The model under review builds one solid part; all positions refer to its coordinate system, in mm. A direction names the side the tool comes from. Round coordinates to 2 decimals unless told otherwise and drop trailing zeros. Write each loop counter-clockwise with the first axis right and the second up, starting at its lowest first coordinate (ties: lowest second). Pieces come first, ordered by that corner, then holes. Notation, with made-up numbers: M 1.25,88.25 L 53.25,88.25 A22 cw 53.25,114.25 Z; hole C 84,-37.5 d2. An arc over 180 degrees is marked long. One line per item, written item: value. Start each with the question number.
1) Take a section at B-B, the plane z = 10. Write out the cut boundary in (x, y).
2) Wall thickness on probe 1 along X at (y, z) = (0, 4.25); probe 2 along Z at (x, y) = (1.5, -5.5): over which ranges is each line inside the solid? List them lowest first.
3) Take a section at C-C, the plane y = 0. Write out the cut boundary in (x, z), and give its area (3 significant figures).
4) Take a section at D-D, the plane z = 4.25. Write out the cut boundary in (x, y), and give its area (3 significant figures).
5) Mouldability with a two-part tool opening along X and no side actions: class faces 3 (the face through (-14.7, 0.65, 5.25)), 4 (the face through (0, -14, 10.644)), 5 (the face through (0, 0, 1.5)) as +X half, -X half, draft (parallel to the pull), parting line (faces both ways), or undercut.
6) For P1, Ø6, axis at x = -9.5, z = 6.5, coming from the +Y side; P2, Ø8, axis at x = 3, y = -8.5, coming from the -Z side; P3, Ø1, axis at y = 1.5, z = 2.5, coming from the -X side, all flat-tipped, find the tip position at first contact; note any pin that passes through.
7) Tool access review of faces 1 (the face through (-10.11, 9.27, 6.01)), 2 (the face through (14.132, -0.047, 6.834)): name each direction out of +Z, -Z, +X, -X, +Y, -Y from which nothing blocks a thin tool from reaching the whole face with its end or side.
8) Take a section at A-A, the plane x = 0. Write out the cut boundary in (y, z), and give its area (3 significant figures).
from build123d import *

# Parameters (mm, degrees)
F2_R          = 14.716
F3_DEPTH      = 1.5
F4_R          = 14.716
F4_R_2        = 13.716
F5_DEPTH      = 9.144
F6_R          = 12.7
F7_DEPTH      = 14.717
F7_DEPTH_BACK = 14.717


with BuildPart() as f3:
    # F2 (on Top) → F3 (new body)
    with BuildSketch(Plane.XY):
        Circle(F2_R)
    extrude(amount=F3_DEPTH)

    # F4 (on face) → F5 (join)
    with BuildSketch(Plane.XY.offset(1.5)):
        Circle(F4_R)
        Circle(F4_R_2, mode=Mode.SUBTRACT)
    extrude(amount=F5_DEPTH)

    # F6 (on Right) → F7 (cut, two sides)
    with BuildSketch(Plane.YZ) as f7_sk:
        with Locations((0, 19.534)):
            Circle(F6_R)
    extrude(amount=-F7_DEPTH, mode=Mode.SUBTRACT)
    extrude(f7_sk.sketch, amount=F7_DEPTH_BACK, mode=Mode.SUBTRACT)


solid = f3.part
Checked values:
1. outline: M -12.09,-8.39 A14.72 ccw 12.09,-8.39 L 10.85,-8.39 A13.72 cw -10.85,-8.39 Z; M -12.09,8.39 L -10.85,8.39 A13.72 cw 10.85,8.39 L 12.09,8.39 A14.72 ccw Z
2. probe 1: x = -14.72 to -13.72, 13.72 to 14.72
2. probe 2: z = 0 to 1.5
3. outline: M -14.72,0 L 14.72,0 L 14.72,6.83 L 13.72,6.83 L 13.72,1.5 L -13.72,1.5 L -13.72,6.83 L -14.72,6.83 Z
3. area: 54.8 mm2
4. outline: C 0,0 d29.43; hole C 0,0 d27.43
4. area: 89.3 mm2
5. face 3: parting line
5. face 4: draft
5. face 5: undercut
6. P1: stops at y = 13.2
6. P2: stops at z = 0
6. P3: stops at x = -14.68
7. face 1: +Z
7. face 2: +Z, +X, -X
8. outline: M -14.72,0 L 14.72,0 L 14.72,10.64 L 13.72,10.64 L 13.72,1.5 L -13.72,1.5 L -13.72,10.64 L -14.72,10.64 Z
8. area: 62.4 mm2
